Answer from the drawing. Dimensions are ordinates in mm from the lowest x, y and z of the part. A direction names the side the tool comes from. Coordinates: 2 decimals unless noted, no trailing zeros. Order: outer loops, then holes, each group sorted by start corner. A loop starts at its lowest first (then second) coordinate and runs counter-clockwise, first axis right, second up. Notation, with made-up numbers: M 42.25,-33.75 L 77.25,-33.75 A16 cw 77.25,-25.75 Z; hole C -25,51 d5. An arc over 180 degrees is marked long. Write each question's results on one line, items separated by ' | '.
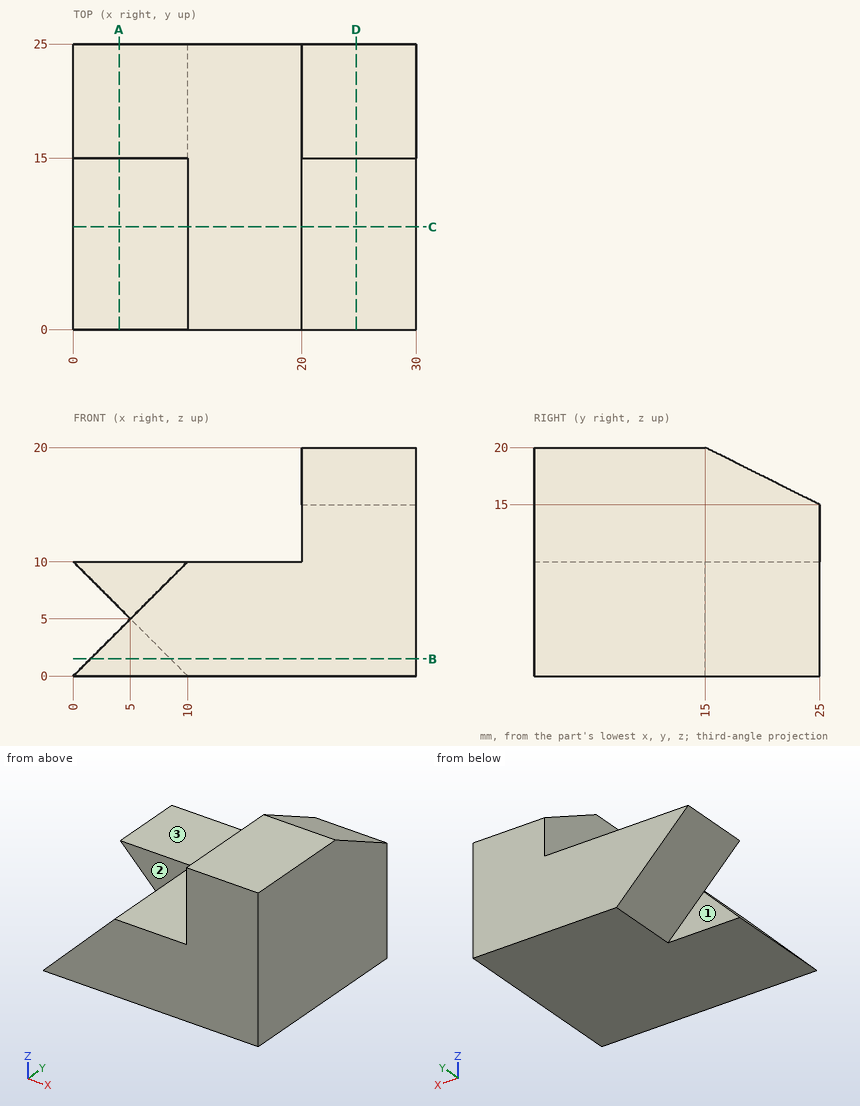
(1) The part is cut by section A-A, the plane x = 4. Write down the section's boundary in (y, z), then the cut area to 4 significant figures.
Conclusion:
outline: M 0,0 L 15,0 L 15,4 L 0,4 Z; M 15,6 L 25,6 L 25,10 L 15,10 Z | area: 100.0 mm²
(2) Given pin 1 (12 mm diameter, centred on x = 7.5, y = 15.5, fed in from +Z); pin 2 (1.5 mm diameter, centred on x = 6.5, z = 2, fed in from +Y); pin 3 (1.5 mm diameter, centred on x = 4, z = 8, fed in from -Y), each flat-ended and moving along its own axis, determine where each tip first touches the part or whether it passes through.
Conclusion:
pin 1: z = 10 | pin 2: y = 15 | pin 3: y = 15
(3) Straight lines are drawn through the part: line 1 (X direction, y = 23.5, z = 12.5); line 2 (Z direction, x = 17.5, y = 9.25); line 3 (Z direction, x = 5.25, y = 17). For each, find the intervals that lie inside material, in ascending order.
Conclusion:
line 1: 20 to 30 | line 2: 0 to 10 | line 3: 4.75 to 10
(4) For the marked faces 1, 2 and 3, determine the directions among +Z, -Z, +X, -X, +Y, -Y from which every point of the face is accessible in a straight line to the end or side of a thin tool.
Conclusion:
face 1: -Z, -X, +Y | face 2: +Z, -X, -Y | face 3: +Z, -X, +Y, -Y
(5) The part is cut by section B-B, the plane z = 1.5. Write down the section's boundary in (x, y).
Conclusion:
outline: M 1.5,0 L 30,0 L 30,25 L 8.5,25 L 8.5,15 L 1.5,15 Z
(6) The part is cut by section D-D, the plane x = 24.75. Write down the section's boundary in (y, z), then the cut area to 3 significant figures.
Conclusion:
outline: M 0,0 L 25,0 L 25,15 L 15,20 L 0,20 Z | area: 475 mm²
(7) The part is cut by section C-C, the plane y = 9. Write down the section's boundary in (x, z), then the cut area to 3 significant figures.
Conclusion:
outline: M 0,0 L 30,0 L 30,20 L 20,20 L 20,10 L 10,10 Z | area: 350 mm²
